from build123d import *

# Parameters (mm, degrees)
SKETCH_1_R      = 2.025
SKETCH_1_R_2    = 2.525
EXTRUDE_1_DEPTH = 2


with BuildPart() as part:
    # 草图1 → 凸台-拉伸1 (new, symmetric)
    with BuildSketch(Plane.XY):
        with BuildLine():
            Line((-14, 4), (14, 4))
            Line((14, 4), (14, -4))
            Line((14, -4), (-22.374938993, -26.284819682))
            ThreePointArc((-22.374938993, -26.284819682), (-28.952100704, -25.103469836), (-28.540142401, -18.433767144))
            Line((-28.540142401, -18.433767144), (-14, -4))
            Line((-14, -4), (-14, 4))
        make_face()
        with Locations((10, 0)):
            Circle(SKETCH_1_R, mode=Mode.SUBTRACT)
        with Locations((-10, 0)):
            Circle(SKETCH_1_R, mode=Mode.SUBTRACT)
        with Locations((-25, -22)):
            Circle(SKETCH_1_R_2, mode=Mode.SUBTRACT)
    extrude(amount=EXTRUDE_1_DEPTH, both=True)


solid = part.part
Design review of the part built by this model. Coordinates are the model's own, in mm. Coordinates: 2 decimals unless noted, no trailing zeros. Order: outer loops, then holes, each group sorted by start corner. A loop starts at its lowest first (then second) coordinate and runs counter-clockwise, first axis right, second up. Notation, with made-up numbers: (77.5, 58) - (128.5, 58) arc R20 cw to (128.5, 75) - close; hole circle Ø1 at (-18, 43). An arc over 180 degrees is marked (long way). Put each result on its own line as item: value.
1) Take a section at C-C, the plane x = -25. Give the boundary of the cut face in (y, z) (3 decimals), and give its area (3 significant figures).
Response values:
outline: (-27.025, -2) - (-24.525, -2) - (-24.525, 2) - (-27.025, 2) - close; (-19.475, -2) - (-14.92, -2) - (-14.92, 2) - (-19.475, 2) - close
area: 28.2 mm²
2) Take a section at A-A, the plane y = 0. Give the boundary of the cut face in (x, z) (3 decimals), and give its area (3 significant figures).
Response values:
outline: (-14, -2) - (-12.025, -2) - (-12.025, 2) - (-14, 2) - close; (-7.975, -2) - (7.975, -2) - (7.975, 2) - (-7.975, 2) - close; (12.025, -2) - (14, -2) - (14, 2) - (12.025, 2) - close
area: 79.6 mm²
3) The part is to be moulded in two halves that separate along X. For faces 1 (the face through (-14, 0, 0)), 2 (the face through (7.977, 0.089, -0.028)), 3 (the face through (-12.023, 0.089, -0.028)), 4 (the face through (0, 4, 0)), say which applies: released by +X, released by -X, zero draft, split by the parting line, or undercut.
Response values:
face 1: released by -X
face 2: undercut
face 3: undercut
face 4: zero draft
4) Take a section at B-B, the plane z = 0.55. Give the boundary of the cut face in (x, y) (3 decimals), and give its area (3 significant figures).
Response values:
outline: (-28.54, -18.434) arc R5.025 ccw to (-22.375, -26.285) - (14, -4) - (14, 4) - (-14, 4) - (-14, -4) - close; hole circle Ø5.05 at (-25, -22); hole circle Ø4.05 at (-10, 0); hole circle Ø4.05 at (10, 0)
area: 626 mm²
5) Insertion check: P1, Ø2.5, axis at x = -10, y = 0, coming from the +Z side; P2, Ø2, axis at y = -9, z = -0.5, coming from the +X side; P3, Ø1.2, axis at y = 0.5, z = 0.5, coming from the -X side; P4, Ø1.5, axis at y = -22, z = 1.5, coming from the +X side. Each pin has a flat end and moves straight along its axis. Give the tip position at first contact, or say it passes through.
Response values:
P1: passes through
P2: stops at x = 7.47
P3: stops at x = -14
P4: stops at x = -14.16
6) Wall thickness on L1, parallel to X at y = 1, z = -1.55; L2, parallel to X at y = 1.5, z = -0.2; L3, parallel to X at y = -23.5, z = 0.4: over which ranges is each line inside the solid? List them lowest first. Write a range as from..to.
Response values:
L1: x = -14..-11.76, -8.24..8.24, 11.76..14
L2: x = -14..-11.36, -8.64..8.64, 11.36..14
L3: x = -29.8..-27.03, -22.97..-17.83
7) Take a section at D-D, the plane y = -21.5. Give the boundary of the cut face in (x, z) (3 decimals).
Response values:
outline: (-30, -2) - (-27.475, -2) - (-27.475, 2) - (-30, 2) - close; (-22.525, -2) - (-14.565, -2) - (-14.565, 2) - (-22.525, 2) - close
